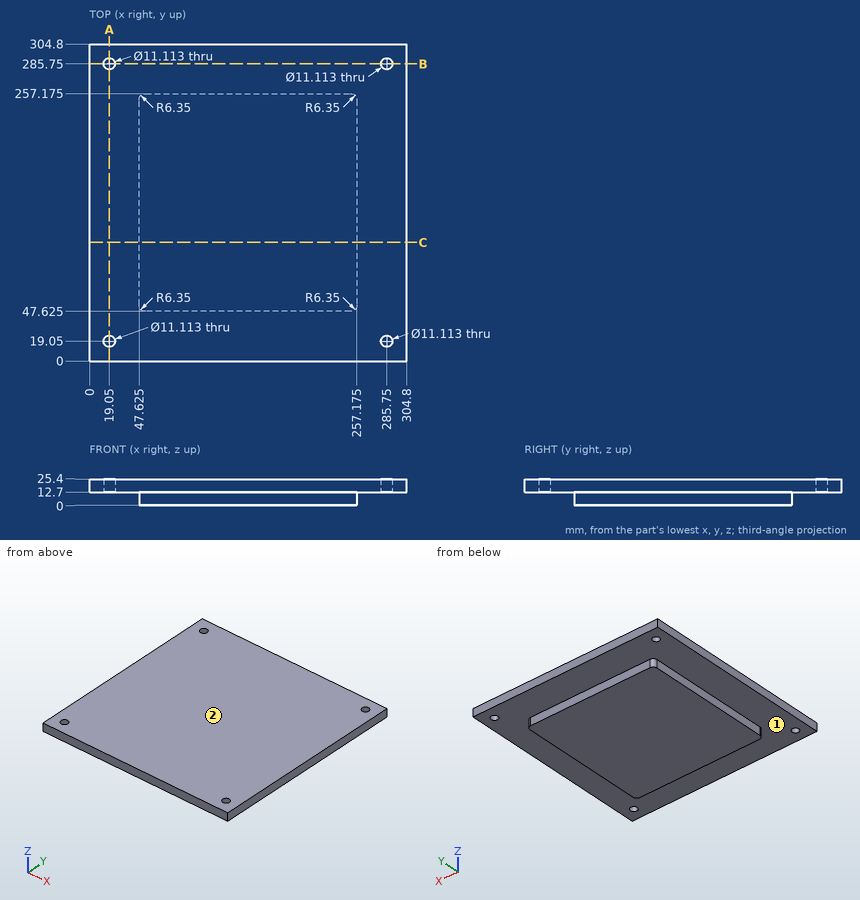
For this review, use the dimensioned drawing (mm, ordinates from the lowest corner) and the shaded views. A direction names the side the tool comes from. Round coordinates to 2 decimals unless told otherwise and drop trailing zeros. Write each loop counter-clockwise with the first axis right and the second up, starting at its lowest first coordinate (ties: lowest second). Pieces come first, ordered by that corner, then holes. Notation, with made-up numbers: M 33,78 L 59,78 A19 ccw 59,93 Z; hole C -13,61.5 d11. An arc over 180 degrees is marked long. Write item = value, one per line. Start each with the question number.
(1) For line 1 along Y through (x, z) = (285.75, 18); line 2 along Z through (x, y) = (156, 27), list the stretches that pass through material, from the lowest coordinate up.
(2) We need section A-A (x = 19.05). Give the boundary of the cut face in (y, z), then the cut area to 3 significant figures.
(3) Clearance check with flat-ended pins moving along their axes: pin 1 Ø6 at (x, y) = (43.5, 45.5) entering from -Z; pin 2 Ø8 at (x, y) = (233.5, 97.5) entering from -Z; pin 3 Ø6.5 at (x, z) = (157, 6) entering from +Y (1 decimal); pin 4 Ø6.5 at (y, z) = (136.5, 6) entering from +X (1 decimal). State where each tip first meets the part, or that it passes through.
(4) For the marked faces 1 and 2, list the 3-axis set-ups (+Z, -Z, +X, -X, +Y, -Y) from which the entire face can be reached by the end or side of a thin tool; tool diameter is ignored.
(5) We need section C-C (y = 114). Give the boundary of the cut face in (x, z) (1 decimal).
Results found:
q1.line_1 = 0 to 13.49, 24.61 to 280.19, 291.31 to 304.8
q1.line_2 = 12.7 to 25.4
q2.outline = M 0,12.7 L 13.49,12.7 L 13.49,25.4 L 0,25.4 Z; M 24.61,12.7 L 280.19,12.7 L 280.19,25.4 L 24.61,25.4 Z; M 291.31,12.7 L 304.8,12.7 L 304.8,25.4 L 291.31,25.4 Z
q2.area = 3,590 mm²
q3.pin_1 = 12.7
q3.pin_2 = 0
q3.pin_3 = 257.2
q3.pin_4 = 257.2
q4.face_1 = -Z
q4.face_2 = +Z, +X, -X, +Y, -Y
q5.outline = M 0,12.7 L 47.6,12.7 L 47.6,0 L 257.2,0 L 257.2,12.7 L 304.8,12.7 L 304.8,25.4 L 0,25.4 Z
